Could you check a few things on this model? Use its own coordinates, in mm. A direction names the side the tool comes from. Coordinates: 2 decimals unless noted, no trailing zeros. Write each loop counter-clockwise with the first axis right and the second up, starting at its lowest first coordinate (ties: lowest second). Pieces come first, ordered by that corner, then holes. Notation, with made-up numbers: M 6,41 L 11,41 A18 cw 11,51 Z; hole C 51.25,18.5 d2. An arc over 180 degrees is marked long. Answer as CSV lines item,"result". Start each with the question number.
Item 1: We'd pull the mould along Y, two halves only. Please class faces 4 (the flat face through (-29, 9.525, 34)), 5 (the flat face through (-36.3, 381, 16.6)), 6 (the flat face through (-28, 1.981, -35)), 7 (the cylindrical face through (-56.3, 4.7, 2.5)): +Y half, -Y half, draft (parallel to the pull), parting line (faces both ways), or undercut.
Item 2: I'm going to push flat-ended pins straight in: P1, Ø1.8, axis at x = 44.71, z = -25.81, coming from the -Y side; P2, Ø8, axis at y = 39, z = 8.5, coming from the -X side; P3, Ø12, axis at x = 15, y = 204.5, coming from the -Z side; P4, Ø10, axis at y = 47, z = 25.5, coming from the +X side. Where does each tip first touch, or does it pass through?
Item 3: On a 3-axis mill with a long thin cutter (end or side, diameter ignored), from which of +Z, -Z, +X, -X, +Y, -Y can I reach the whole of each face in a straight line? I mean faces 1 (the cylindrical face through (-9.6, 0.98, -43.23)), 2 (the cylindrical face through (-10.167, 380.023, -45.786)), 3 (the flat face through (29.4, 31.75, 29.4)). Say none if no direction works.
Item 4: If I drill on line 1 along Z through (x, y) = (0, 4.75); line 2 along Y through (x, z) = (-39, 29.5) (3 decimals); line 3 along Y through (x, z) = (8.5, 43.5), over which ranges is the centre line in solid material (lowest first)? Write a range as [from, to].
Item 5: Suppose I cut it at A-A, the plane y = 67.5. Write out the boundary of the cut face in (x, z) (3 decimals).
```python
from build123d import *

# Parameters (mm, degrees)
SKETCH2_R               = 41.275
SKETCH2_R_2             = 38.1
BASE_CYLINDER_DEPTH     = 381
SKETCH3_R               = 56.35625
SKETCH3_R_2             = 38.1
AFT_FLANGE_DEPTH        = 9.525
SKETCH34_R              = 39.75
TEMPERATUREINSERT_DEPTH = 28.575
SKETCH6_R               = 46.9011
SKETCH6_R_2             = 44.2849
AFT_O_RING_DEPTH        = 1.9812
SKETCH33_R              = 44.45
SKETCH33_R_2            = 41.275
CRITICALBOSS_DEPTH      = 22.225
BOLT_CIRCLE_D           = 2.2606
BOLT_CIRCLE_DEPTH       = 381
HOLE1_D                 = 2.38125
HOLE1_DEPTH             = 381
HOLE1_CBORE_D           = 4.7625
HOLE1_CBORE_DEPTH       = 4.7625


with BuildPart() as part:
    # Sketch2 → Base Cylinder (new body)
    with BuildSketch(Plane(origin=(0, 0, 0), x_dir=(1, 0, 0), z_dir=(0, 1, 0))):
        Circle(SKETCH2_R)
        Circle(SKETCH2_R_2, mode=Mode.SUBTRACT)
    extrude(amount=BASE_CYLINDER_DEPTH)

    # Sketch3 → Aft Flange (add)
    with BuildSketch(Plane.XZ):
        Circle(SKETCH3_R)
        Circle(SKETCH3_R_2, mode=Mode.SUBTRACT)
    aft_flange = extrude(amount=-AFT_FLANGE_DEPTH)

    # Sketch34 → TemperatureInsert (cut)
    with BuildSketch(Plane.XZ):
        Circle(SKETCH34_R)
    temperatureinsert = extrude(amount=-TEMPERATUREINSERT_DEPTH, mode=Mode.SUBTRACT)

    # Sketch6 → Aft O-Ring (cut)
    with BuildSketch(Plane.XZ):
        Circle(SKETCH6_R)
        Circle(SKETCH6_R_2, mode=Mode.SUBTRACT)
    aft_o_ring = extrude(amount=-AFT_O_RING_DEPTH, mode=Mode.SUBTRACT)

    # Sketch33 → CriticalBoss (add)
    with BuildSketch(Plane(origin=(0, 9.525, 0), x_dir=(1, 0, 0), z_dir=(0, 1, 0))):
        Circle(SKETCH33_R)
        Circle(SKETCH33_R_2, mode=Mode.SUBTRACT)
    criticalboss = extrude(amount=CRITICALBOSS_DEPTH)

    # Bolt Circle
    with Locations(Plane(origin=(0, 0, 0), x_dir=(-1, 0, 0), z_dir=(0, -1, 0))):
        with Locations((-25.81275, -44.708994483), (-44.708994483, -25.81275), (-51.6255, 0), (-44.708994483, 25.81275), (-25.81275, 44.708994483), (0, 51.6255), (25.81275, 44.708994483), (44.708994483, 25.81275), (51.6255, 0), (44.708994483, -25.81275), (25.81275, -44.708994483), (0, -51.6255)):
            bolt_circle = Hole(BOLT_CIRCLE_D / 2, depth=BOLT_CIRCLE_DEPTH)

    # Hole1
    with Locations(Plane(origin=(0, 0, 0), x_dir=(-1, 0, 0), z_dir=(0, -1, 0))):
        with Locations((49.866403745, 13.361662613), (-49.866403745, -13.361662613)):
            hole1 = CounterBoreHole(HOLE1_D / 2, HOLE1_CBORE_D / 2, HOLE1_CBORE_DEPTH, depth=HOLE1_DEPTH)

    # Mirror1: Aft Flange, TemperatureInsert, Aft O-Ring, CriticalBoss, Bolt Circle, Hole1 across plane
    add(aft_flange.mirror(Plane.ZX.offset(190.5)))
    add(temperatureinsert.mirror(Plane.ZX.offset(190.5)), mode=Mode.SUBTRACT)
    add(aft_o_ring.mirror(Plane.ZX.offset(190.5)), mode=Mode.SUBTRACT)
    add(criticalboss.mirror(Plane.ZX.offset(190.5)))
    add(bolt_circle.mirror(Plane.ZX.offset(190.5)), mode=Mode.SUBTRACT)
    add(hole1.mirror(Plane.ZX.offset(190.5)), mode=Mode.SUBTRACT)


solid = part.part
```
Ans:
1,face 4,"undercut"
1,face 5,"+Y half"
1,face 6,"-Y half"
1,face 7,"draft"
2,P1,"passes through"
2,P2,"stops at x = -41.03"
2,P3,"stops at z = -40.28"
2,P4,"stops at x = 35.82"
3,face 1,"-Y"
3,face 2,"+Y"
3,face 3,"none"
4,line 1,"z = [-56.36, -52.76], [-50.5, -39.75], [39.75, 50.5], [52.76, 56.36]"
4,line 2,"y = [0, 9.525], [371.475, 381]"
4,line 3,"y = [1.98, 31.75], [349.25, 379.02]"
5,outline,"C 0,0 d82.55; hole C 0,0 d76.2"
